Input: part model. Units: mm. Frame: model coordinates. A direction names the side the tool comes from. Give positions to 0.01 mm unless a question says otherwise; leave off trailing zeros. Loops run counter-clockwise (first coordinate to the right, second up) from the corner with the lowest first, then second, coordinate; pieces in that order, holes last. Notation, with made-up numbers: M 85.25,2 L 112.25,2 A29 ccw 112.25,41 Z; hole C -31.75,-20 d5. An arc over 180 degrees is marked long. Return JSON: item names as keys, results as strings. Group by question number.
```python
from build123d import *

# Parameters (mm, degrees)
F0_R     = 17.5
F0_W     = 10
F0_H     = 30
F0_W_2   = 8
F0_H_2   = 15
F1_DEPTH = 15
F2_R     = 2.1


with BuildPart() as f1:
    # F0 (on Top) → F1 (new body)
    with BuildSketch(Plane.XY):
        Polygon((29.2293787445, 29.4917059159), (-113.5933991075, 29.4917059159), (-113.5933991075, 4.4917059159), (-103.5933991075, 4.4917059159), (-93.5933991075, 4.4917059159), (-85.5933991075, 4.4917059159), (-75.5933991075, 4.4917059159), (-61.5933991075, 4.4917059159), (29.2293787445, 4.4917059159), align=None)
        with BuildLine():
            ThreePointArc((29.2293787445, 4.4917059159), (96.9211208211, 16.9917059159), (29.2293787445, 29.4917059159))
            Line((29.2293787445, 29.4917059159), (29.2293787445, 4.4917059159))
        make_face()
        with Locations((61.9211208211, 16.9917059159)):
            Circle(F0_R, mode=Mode.SUBTRACT)
        with Locations((-108.5933991075, -10.5082940841)):
            Rectangle(F0_W, F0_H)
        Polygon((-68.5933991075, -10.5082940841), (-61.5933991075, 4.4917059159), (-75.5933991075, 4.4917059159), align=None)
        with Locations((-89.5933991075, -3.0082940841)):
            Rectangle(F0_W_2, F0_H_2)
    extrude(amount=F1_DEPTH)

    # F2
    f2_edges = [f1.edges().sort_by_distance(p)[0] for p in [
        (-113.593399, 1.991706, 0),
        (-113.593399, 29.491706, 7.5),
        (-113.593399, 1.991706, 15),
        (-113.593399, -25.508294, 7.5),
        (-42.18201, 29.491706, 0),
        (-16.18201, 4.491706, 15),
        (-42.18201, 29.491706, 15),
        (96.921121, 16.991706, 15),
        (96.921121, 16.991706, 0),
        (-65.093399, -3.008294, 15),
        (-85.593399, -3.008294, 15),
        (-80.593399, 4.491706, 15),
        (-72.093399, -3.008294, 15),
        (-89.593399, -10.508294, 15),
        (-93.593399, 4.491706, 7.5),
        (-103.593399, -10.508294, 15),
        (-93.593399, -10.508294, 7.5),
        (-89.593399, -10.508294, 0),
        (-72.093399, -3.008294, 0),
        (-68.593399, -10.508294, 7.5),
        (-98.593399, 4.491706, 15),
        (44.421121, 16.991706, 0),
        (-93.593399, -3.008294, 15),
    ]]
    fillet(f2_edges, radius=F2_R)


solid = f1.part
```
Item 1: First-contact query: pin 1 Ø6 at (x, z) = (48, 3) entering from +Y; pin 2 Ø3 at (y, z) = (10.5, 7.5) entering from +X; pin 3 Ø8.5 at (x, z) = (-22, 7.5) entering from +Y; pin 4 Ø6 at (x, y) = (20, 3) entering from -Z. Flat tips, straight axial feed; report the tip coordinate or a pass-through.
Item 2: Reachability of faces 1 (the face through (-93.593, -3, 6)), 2 (the face through (-40, 29.492, 7)), 3 (the face through (-64.362, -0.025, 14.369)) from +Z, -Z, +X, -X, +Y, -Y: full face, straight path, thin tool, end or side. Return the list, or none.
Item 3: Material intervals for line 1 (X direction, y = -12, z = 5.25); line 2 (X direction, y = 18, z = 12.25); line 3 (Y direction, x = 23.5, z = 2.5), sorted ascending. Write a range as from..to.
Item 4: Section B-B, the plane x = 17. Return loops of the section in (y, z), then the cut area to 3 significant figures.
Item 5: Pull-direction query (X, two-part tool) for faces 4 (the face through (-73.08, -0.89, 7.42)), 5 (the face through (-1, 12, 15)); classes: pulls with the +X half, pulls with the -X half, needs draft (parallel to the pull), parting line crosses it, or undercut.
Item 6: Section A-A, the plane z = 8.75. Return loops of the section in (x, y).
Answer below:
{
 "1": {"pin 1": "y = 50.24", "pin 2": "x = 96.56", "pin 3": "y = 29.49", "pin 4": "z = 0"},
 "2": {"face 1": "+Z, -Z, -Y", "face 2": "+Z, -Z, -X, +Y", "face 3": "+Z, -Y"},
 "3": {"line 1": "-113.59..-103.59, 42.31..81.53", "line 2": "-113.59..44.45, 79.39..96.91", "line 3": "4.49..29.49"},
 "4": {"outline": "M 4.49,0 L 27.39,0 A2.1 ccw 29.49,2.1 L 29.49,12.9 A2.1 ccw 27.39,15 L 6.59,15 A2.1 ccw 4.49,12.9 Z", "area": "372 mm^2"},
 "5": {"face 4": "undercut", "face 5": "needs draft"},
 "6": {"outline": "M -113.59,-23.41 A2.1 ccw -111.49,-25.51 L -103.59,-25.51 L -103.59,4.49 L -95.69,4.49 A2.1 cw -93.59,2.39 L -93.59,-8.41 A2.1 ccw -91.49,-10.51 L -85.59,-10.51 L -85.59,4.49 L -75.59,4.49 L -70.5,-6.43 A2.1 ccw -66.69,-6.43 L -61.59,4.49 L 29.23,4.49 A35 ccw long 29.23,29.49 L -111.49,29.49 A2.1 ccw -113.59,27.39 Z; hole C 61.92,16.99 d35"}
}
